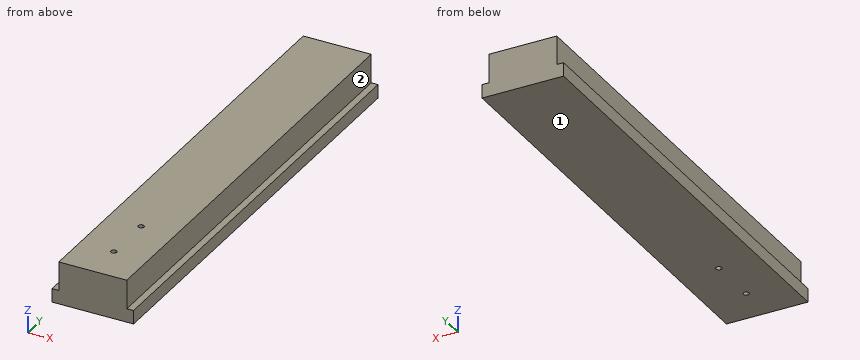
from build123d import *

# Parameters (mm, degrees)
F1_DEPTH = 127
F3_DEPTH = 25.4


with BuildPart() as f1:
    # F0 (on Front) → F1 (new body)
    with BuildSketch(Plane.XZ):
        Polygon((-11.43, 0), (0, 0), (11.43, 0), (11.43, 3.829304), (9.525, 3.829304), (9.525, 11.938), (-9.525, 11.938), (-9.525, 3.829304), (-11.43, 3.829304), align=None)
    extrude(amount=F1_DEPTH)

    # F2 (on face) → F3 (cut)
    with BuildSketch(Plane.XY.offset(11.938)):
        with BuildLine():
            ThreePointArc((0.79375, -101.8351912498), (0.5612660076, -101.2739252423), (0, -101.0414412498))
            Line((0, -101.0414412498), (0, -102.6289412498))
            ThreePointArc((0, -102.6289412498), (0.5612660076, -102.3964572574), (0.79375, -101.8351912498))
        make_face()
        with BuildLine():
            Line((0, -102.6289412498), (0, -101.0414412498))
            ThreePointArc((0, -101.0414412498), (-0.79375, -101.8351912498), (0, -102.6289412498))
        make_face()
        with BuildLine():
            Line((0, -116.8494993567), (0, -115.2619993567))
            ThreePointArc((0, -115.2619993567), (-0.79375, -116.0557493567), (0, -116.8494993567))
        make_face()
        with BuildLine():
            ThreePointArc((0.79375, -116.0557493567), (0.5612660076, -115.4944833492), (0, -115.2619993567))
            Line((0, -115.2619993567), (0, -116.8494993567))
            ThreePointArc((0, -116.8494993567), (0.5612660076, -116.6170153643), (0.79375, -116.0557493567))
        make_face()
    extrude(amount=-F3_DEPTH, mode=Mode.SUBTRACT)


solid = f1.part
CAD build for the part. Positions are in the model's coordinates, mm. Face numbers are marked on the shaded views. A direction names the side the tool comes from. Coordinates: 2 decimals unless noted, no trailing zeros. Order: outer loops, then holes, each group sorted by start corner. A loop starts at its lowest first (then second) coordinate and runs counter-clockwise, first axis right, second up. Notation, with made-up numbers: (48.25, -25.5) -> (76.25, -25.5) arc R20 ccw to (76.25, 9.5) -> close; hole circle Ø10 at (2.5, 42.25). An arc over 180 degrees is marked (long way). Answer in a Markdown table with one row per item.
1) Band-saw the part on B-B (y = -44.5). List the corners of the cut face in (x, z) (3 decimals).
Check values:
| item | result |
|---|---|
| outline | (-11.43, 0) -> (11.43, 0) -> (11.43, 3.829) -> (9.525, 3.829) -> (9.525, 11.938) -> (-9.525, 11.938) -> (-9.525, 3.829) -> (-11.43, 3.829) -> close |
2) Band-saw the part on A-A (z = 5). List the corners of the cut face in (x, y) (1 decimal), and give its area (3 significant figures).
Check values:
| item | result |
|---|---|
| outline | (-9.5, -127) -> (9.5, -127) -> (9.5, 0) -> (-9.5, 0) -> close; hole circle Ø1.6 at (0, -116.1); hole circle Ø1.6 at (0, -101.8) |
| area | 2,420 mm2 |
3) Drill centre lines: line 1 (X direction, y = -79, z = 7.25) (3 decimals); line 2 (Y direction, x = 0.25, z = 5.5); line 3 (X direction, y = -102.5, z = 3). Where is each one in solid material? Low to high.
Check values:
| item | result |
|---|---|
| line 1 | -9.525 to 9.525 |
| line 2 | -127 to -116.81, -115.3 to -102.59, -101.08 to 0 |
| line 3 | -11.43 to -0.43, 0.43 to 11.43 |
4) Flat gauge pins, fed straight in: P1, Ø0.6, axis at x = -10.5, y = -65, coming from the +Z side; P2, Ø2.5, axis at y = -75.5, z = 8, coming from the +X side (3 decimals). Where does each tip first touch, or does it go through?
Check values:
| item | result |
|---|---|
| P1 | z = 3.83 |
| P2 | x = 9.525 |
5) Which spindle directions (+Z, -Z, +X, -X, +Y, -Y) get a long thin tool onto all of the face, cutting with end or side? Do the marked faces 1 and 2. Say none if no direction does.
Check values:
| item | result |
|---|---|
| face 1 | -Z, +X, -X, +Y, -Y |
| face 2 | +Z, +X, +Y, -Y |
